Print and shaded views of the part. All mm, measured from the part's lowest x, y and z. A direction names the side the tool comes from. Coordinates: 2 decimals unless noted, no trailing zeros. Order: outer loops, then holes, each group sorted by start corner. A loop starts at its lowest first (then second) coordinate and runs counter-clockwise, first axis right, second up. Notation, with made-up numbers: (87.5, 73.5) -> (93.5, 73.5) arc R7 cw to (93.5, 82.5) -> close; hole circle Ø3 at (7.5, 37). An arc over 180 degrees is marked (long way). Return JSON: item names as keys, results as strings. Group by question number.
1) Cut at C-C (x = 7.5). Write the cut outline in (y, z).
2) Flat gauge pins, fed straight in: pin 1 (4 mm diameter, centred on x = 2.5, y = 7.5, fed in from +Z); pin 2 (4 mm diameter, centred on y = 5.5, z = 6, fed in from +X); pin 3 (1.5 mm diameter, centred on x = 9.5, y = 8, fed in from -Z); pin 4 (1.8 mm diameter, centred on x = 2, y = 9, fed in from -Z). Where does each tip first touch, or does it go through?
3) Which spindle directions (+Z, -Z, +X, -X, +Y, -Y) get a long thin tool onto all of the face, cutting with end or side? Do the marked faces 1, 2, 3 and 4. Say none if no direction does.
4) Cut at B-B (y = 4.75). Write the cut outline in (x, z).
5) Cut at D-D (y = 3). Write the cut outline in (x, z).
6) Cut at A-A (z = 5). Write the cut outline in (x, y).
7) Probe line 1 (Z direction, x = 7.5, y = 3.85); line 2 (X direction, y = 7.5, z = 7.5); line 3 (Y direction, x = 1.75, z = 3.5). List the from-to ranges inside material, lowest first.
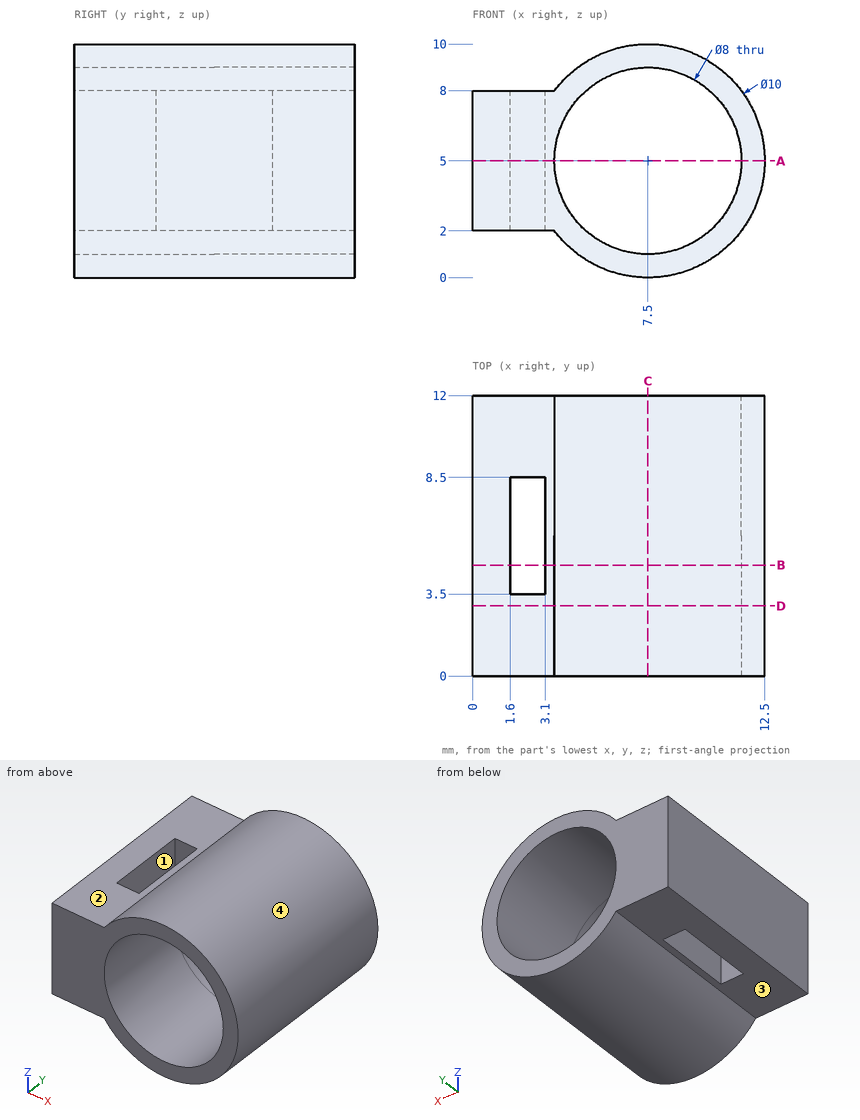
Answers below:
{
 "1": {"outline": "(0, 0) -> (12, 0) -> (12, 1) -> (0, 1) -> close; (0, 9) -> (12, 9) -> (12, 10) -> (0, 10) -> close"},
 "2": {"pin 1": "stops at z = 9", "pin 2": "stops at x = 12.5", "pin 3": "stops at z = 0.16", "pin 4": "stops at z = 2"},
 "3": {"face 1": "+Z, -Z", "face 2": "+Z, -X, +Y, -Y", "face 3": "-Z, -X, +Y, -Y", "face 4": "+Y, -Y"},
 "4": {"outline": "(0, 2) -> (1.6, 2) -> (1.6, 8) -> (0, 8) -> close; (3.1, 2) -> (3.5, 2) arc R5 ccw (long way) to (3.5, 8) -> (3.1, 8) -> close; hole circle Ø8 at (7.5, 5)"},
 "5": {"outline": "(0, 2) -> (3.5, 2) arc R5 ccw (long way) to (3.5, 8) -> (0, 8) -> close; hole circle Ø8 at (7.5, 5)"},
 "6": {"outline": "(0, 0) -> (3.5, 0) -> (3.5, 12) -> (0, 12) -> close; (11.5, 0) -> (12.5, 0) -> (12.5, 12) -> (11.5, 12) -> close; hole (1.6, 3.5) -> (3.1, 3.5) -> (3.1, 8.5) -> (1.6, 8.5) -> close"},
 "7": {"line 1": "z = 0 to 1, 9 to 10", "line 2": "x = 0 to 1.6, 3.1 to 4.38, 10.62 to 11.83", "line 3": "y = 0 to 3.5, 8.5 to 12"}
}
